CAD build for the part. Positions are in the model's coordinates, mm. Face numbers are marked on the shaded views. Round coordinates to 2 decimals unless told otherwise and drop trailing zeros. Loops run counter-clockwise (first coordinate to the right, second up) from the corner with the lowest first, then second, coordinate; pieces in that order, holes last.
```python
from build123d import *

# Parameters (mm, degrees)
F0_W     = 50.8
F0_H     = 88.9
F1_DEPTH = 3.175
F2_W     = 3.175
F2_H     = 42.8625
F3_DEPTH = 3.175
F4_DEPTH = 3.175


with BuildPart() as f1:
    # F0 (on Front) → F1 (new body)
    with BuildSketch(Plane.XZ):
        Rectangle(F0_W, F0_H)
    extrude(amount=F1_DEPTH)

    # F2 (on face) → F3 (cut)
    with BuildSketch(Plane.XZ.offset(3.175)):
        with Locations((0, -23.309385)):
            Rectangle(F2_W, F2_H)
    extrude(amount=-F3_DEPTH, mode=Mode.SUBTRACT)

    # F2 (on face) → F4 (cut)
    with BuildSketch(Plane.XZ.offset(3.175)):
        with Locations((0, -23.309385)):
            Rectangle(F2_W, F2_H)
    extrude(amount=-F4_DEPTH, mode=Mode.SUBTRACT)


solid = f1.part
```
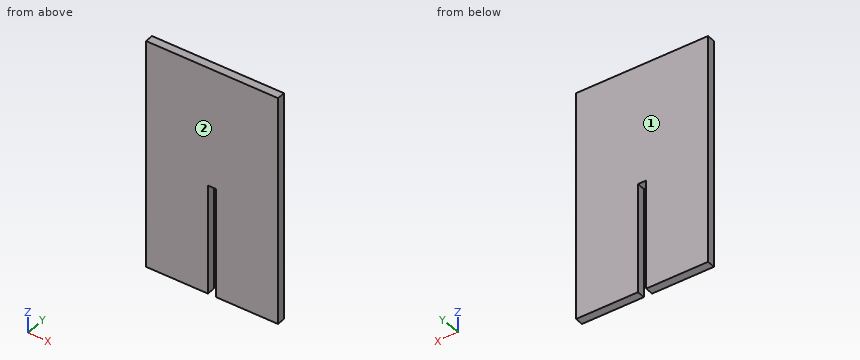
Item 1: Cut at B-B, the plane y = -2.1. Give the cut face in (x, z).
Answers follow:
outline: (-25.4, -44.45) - (-1.59, -44.45) - (-1.59, -1.88) - (1.59, -1.88) - (1.59, -44.45) - (25.4, -44.45) - (25.4, 44.45) - (-25.4, 44.45) - close
Item 2: Cut at C-C, the plane x = 0. Give the cut face in (y, z) (3 decimals), plus the area to 3 significant figures.
Answers follow:
outline: (-3.175, -1.878) - (0, -1.878) - (0, 44.45) - (-3.175, 44.45) - close
area: 147 mm2
Item 3: Probe line 1 (X direction, y = -2.3, z = -8); line 2 (Z direction, x = 1, y = -2.9). List the from-to ranges inside material, lowest first.
Answers follow:
line 1: x = -25.4 to -1.59, 1.59 to 25.4
line 2: z = -1.88 to 44.45
Item 4: Two-plate mould, pull along Y, no slides. Class the marked faces 1 and 2: released by +Y, released by -Y, zero draft, split by the parting line, or undercut.
Answers follow:
face 1: released by +Y
face 2: released by -Y
Item 5: Cut at A-A, the plane z = -25. Give the cut face in (x, y) (1 decimal), plus the area to 3 significant figures.
Answers follow:
outline: (-25.4, -3.2) - (-1.6, -3.2) - (-1.6, 0) - (-25.4, 0) - close; (1.6, -3.2) - (25.4, -3.2) - (25.4, 0) - (1.6, 0) - close
area: 151 mm2
Item 6: Flat gauge pin, fed straight in: P1, Ø1, axis at x = 0.5, y = -2.5, coming from the -Z side. Where does the tip first touch, or does it go through?
Answers follow:
P1: stops at z = -1.88
